For this review, take the finished solid that the model builds, in its own axes (mm). A direction names the side the tool comes from. Give positions to 0.01 mm unless a question says otherwise; leave off trailing zeros. Loops run counter-clockwise (first coordinate to the right, second up) from the corner with the lowest first, then second, coordinate; pieces in that order, holes last. Notation, with made-up numbers: (12, 30) - (64, 30) arc R9 cw to (64, 36) - close; hole circle Ø7 at (-23.5, 39). An arc over 180 degrees is marked (long way). Answer as CSV lines item,"result".
Autodesk Inventor part; units mm, degrees
ref_plane "YZ Plane" through (0, 0, 0) normal (1, 0, 0) x (0, 1, 0)
ref_plane "XZ Plane" through (0, 0, 0) normal (0, 1, 0) x (-1, 0, 0)
ref_plane "XY Plane" through (0, 0, 0) normal (0, 0, 1) x (1, 0, 0)
sketch "スケッチ1" plane through (0, 0, 0) normal (0, 0, 1) x (1, 0, 0)
  line L0 (7.5, 7.5) -> (-7.5, 7.5)
  line L1 (-7.5, 7.5) -> (-7.5, -7.5)
  line L2 (-7.5, -7.5) -> (7.5, -7.5)
  line L3 (7.5, -7.5) -> (7.5, 7.5)
  line L4 (7.5, 7.5) -> (-7.5, -7.5) construction
  line L5 (-7.5, 7.5) -> (7.5, -7.5) construction
  line L6 (-6.5, 6.5) -> (6.5, 6.5)
  line L7 (6.5, 6.5) -> (6.5, -6.5)
  line L8 (6.5, -6.5) -> (-6.5, -6.5)
  line L9 (-6.5, -6.5) -> (-6.5, 6.5)
  point P0 (0, 0)
  dimension "d0" = 15
  dimension "d1" = 15
  dimension "d2" = 1
extrude "押し出し1" add sketch "スケッチ1" along normal blind 520
sketch "スケッチ2" plane through (-7.5, 7.5, 0) normal (0, 1, 0) x (1, 0, 0)
  circle A0 centre (7.5, -10) radius 1.6
  circle A1 centre (7.5, -20) radius 1.6
  circle A2 centre (7.5, -30) radius 1.6
  line L0 (15, 0) -> (0, 0)
  circle A3 centre (7.5, -490) radius 1.6
  circle A4 centre (7.5, -500) radius 1.6
  circle A5 centre (7.5, -510) radius 1.6
  line L1 (15, -520) -> (0, -520)
  point P0 (7.5, 0)
  point P1 (7.5, 0)
  dimension "d5" = 3.2
  dimension "d6" = 3.2
  dimension "d7" = 3.2
  dimension "d8" = 10
  dimension "d9" = 10
  dimension "d10" = 10
  dimension "d11" = 3.2
  dimension "d12" = 3.2
  dimension "d13" = 3.2
  dimension "d14" = 10
  dimension "d15" = 10
  dimension "d16" = 10
extrude "押し出し2" cut sketch "スケッチ2" against normal through all
properties part number "プレート保持_角柱3" material "アルミニウム 6061"
1) Consider section A-A on z = 397.5. Write out the cut boundary in (x, y), and give its area (3 significant figures).
From the geometry:
outline,"(-7.5, -7.5) - (7.5, -7.5) - (7.5, 7.5) - (-7.5, 7.5) - close; hole (-6.5, -6.5) - (6.5, -6.5) - (6.5, 6.5) - (-6.5, 6.5) - close"
area,"56.0 mm^2"
2) Machinability: for faces 1 (the flat face through (-6.5, 0, 256)), 2 (the flat face through (-7, 0, 0)), which of the approach directions +Z, -Z, +X, -X, +Y, -Y give a long, thin tool a straight path to every point of the face, cutting with its end or side? Answer none if there is none.
From the geometry:
face 1,"+Z, -Z"
face 2,"-Z, +X, -X, +Y, -Y"
3) Consider section B-B on y = 3. Write out the cut boundary in (x, z), and give its area (3 significant figures).
From the geometry:
outline,"(-7.5, 0) - (-6.5, 0) - (-6.5, 520) - (-7.5, 520) - close; (6.5, 0) - (7.5, 0) - (7.5, 520) - (6.5, 520) - close"
area,"1,040 mm^2"
4) Draft analysis for pull direction Y (two halves, no side actions). For faces 3 (the flat face through (0, 7.5, 256)), 4 (the flat face through (7.5, 0, 256)), 5 (the flat face through (0, -6.5, 256)), state which applies: pulls with the +Y half, pulls with the -Y half, needs draft (parallel to the pull), parting line crosses it, or undercut.
From the geometry:
face 3,"pulls with the +Y half"
face 4,"needs draft"
face 5,"undercut"
5) Insertion check: P1, Ø4, axis at x = 0, z = 30, coming from the -Y side. The pin has a flat end and moves straight along its axis. Give the tip position at first contact, or say it passes through.
From the geometry:
P1,"stops at y = -7.5"
6) Wall thickness on line 1 (Y direction, x = -1.5, z = 56.5); line 2 (X direction, y = -7.2, z = 30): over which ranges is each line inside the solid? List them lowest first. Write a range as from..to.
From the geometry:
line 1,"y = -7.5..-6.5, 6.5..7.5"
line 2,"x = -7.5..-1.6, 1.6..7.5"
